Read the model definition and answer for the solid it produces. Units are mm, in the model's axes. A direction names the side the tool comes from. Coordinates: 2 decimals unless noted, no trailing zeros. Write each loop counter-clockwise with the first axis right and the second up, starting at its lowest first coordinate (ties: lowest second). Pieces come first, ordered by that corner, then holes.
1) The part is cut by section C-C (z = -9). Determine the outline of the cut face in (x, y), then the cut area to 3 significant figures.
2) Which of the six approach directions +Z, -Z, +X, -X, +Y, -Y give full straight-line access (tool end or side, diameter ignored) to faces 4 (the face through (30, 43, 0)), 5 (the face through (-35.18, 9.13, 0.96)), 6 (the face through (27.5, 163.4, -0.1))?
3) The part is cut by section A-A (y = 158). Determine the outline of the cut face in (x, z), then the cut area to 3 significant figures.
4) Find the intervals of material crossed by line 1 (Z direction, x = 37, y = 14); line 2 (X direction, y = 5.75, z = -25); line 3 (Y direction, x = 30.5, z = -20.5), in increasing order.
5) The part is cut by section D-D (x = -37). Determine the outline of the cut face in (y, z), then the cut area to 3 significant figures.
6) Determine the mould class of faces 1 (the face through (-32.5, 121, 0)), 2 (the face through (34, 18, 0)), 3 (the face through (25.4, 153.76, 0.17)) for opening direction X: +X half, -X half, draft (parallel to the pull), parting line (faces both ways), or undercut.
7) The part is cut by section B-B (x = 37.5). Determine the outline of the cut face in (y, z).
8) Each of these flat-tipped pins is pushed along its axis until it touches: pin 1 Ø8 at (x, z) = (37.5, 0) entering from -Y; pin 2 Ø5 at (y, z) = (72.5, 22.5) entering from +X; pin 3 Ø25 at (y, z) = (32.5, 0) entering from +X; pin 4 Ø6 at (x, z) = (-37.5, -25) entering from -Y. Where does it stop, or does it pass through?
from build123d import *

# Parameters (mm, degrees)
SKIZZE1_W                            = 90
SKIZZE1_H                            = 172
AUFSATZ_LINEAR_AUSTRAGEN1_DEPTH      = 65
SKIZZE2_W                            = 15
SKIZZE2_H                            = 154
SCHNITT_LINEAR_AUSTRAGEN1_DEPTH      = 190.298705754
SKIZZE3_W                            = 65
SKIZZE3_H                            = 104
AUFSATZ_LINEAR_AUSTRAGEN2_DEPTH      = 2.5
SKIZZE4_W                            = 15
SKIZZE4_H                            = 154
SCHNITT_LINEAR_AUSTRAGEN2_DEPTH      = 190.298705754
SKIZZE5_W                            = 65
SKIZZE5_H                            = 104
AUFSATZ_LINEAR_AUSTRAGEN3_DEPTH      = 2.5
F_6_6_6_6_DURCHMESSER_BOHRUNG1_D     = 6.6
F_6_6_6_6_DURCHMESSER_BOHRUNG1_DEPTH = 172
BOHRUNG1_D                           = 5.02
BOHRUNG1_DEPTH                       = 172
F_6_6_6_6_DURCHMESSER_BOHRUNG2_D     = 6.6
BOHRUNG2_D                           = 5.02
F_5_0_5_DURCHMESSER_BOHRUNG1_D       = 5
F_5_0_5_DURCHMESSER_BOHRUNG1_DEPTH   = 17
F_5_0_5_DURCHMESSER_BOHRUNG1_TIP     = 1.502151548


with BuildPart() as part:
    # Skizze1 → Aufsatz-Linear austragen1 (new body)
    with BuildSketch(Plane(origin=(0, 0, -32.5), x_dir=(-1, 0, 0), z_dir=(0, 0, -1))):
        with Locations((0, 86)):
            Rectangle(SKIZZE1_W, SKIZZE1_H)
    extrude(amount=-AUFSATZ_LINEAR_AUSTRAGEN1_DEPTH)

    # Skizze2 → Schnitt-Linear austragen1 (cut, through all)
    with BuildSketch(Plane.XY.offset(32.5)):
        with Locations((-37.5, 95)):
            Rectangle(SKIZZE2_W, SKIZZE2_H)
    extrude(amount=-SCHNITT_LINEAR_AUSTRAGEN1_DEPTH, mode=Mode.SUBTRACT)

    # Skizze3 → Aufsatz-Linear austragen2 (add)
    with BuildSketch(Plane.ZY.offset(30)):
        with Locations((0, 120)):
            Rectangle(SKIZZE3_W, SKIZZE3_H)
    extrude(amount=AUFSATZ_LINEAR_AUSTRAGEN2_DEPTH)

    # Skizze4 → Schnitt-Linear austragen2 (cut, through all)
    with BuildSketch(Plane.XY.offset(32.5)):
        with Locations((37.5, 95)):
            Rectangle(SKIZZE4_W, SKIZZE4_H)
    extrude(amount=-SCHNITT_LINEAR_AUSTRAGEN2_DEPTH, mode=Mode.SUBTRACT)

    # Skizze5 → Aufsatz-Linear austragen3 (add)
    with BuildSketch(Plane(origin=(30, 0, 0), x_dir=(0, 0, -1), z_dir=(1, 0, 0))):
        with Locations((0, 120)):
            Rectangle(SKIZZE5_W, SKIZZE5_H)
    extrude(amount=AUFSATZ_LINEAR_AUSTRAGEN3_DEPTH)

    # Ø6.6 (6.6) Durchmesser Bohrung1
    with Locations(Plane(origin=(0, 0, 0), x_dir=(-1, 0, 0), z_dir=(0, -1, 0))):
        with Locations((37.5, -25), (37.5, 25)):
            Hole(F_6_6_6_6_DURCHMESSER_BOHRUNG1_D / 2, depth=F_6_6_6_6_DURCHMESSER_BOHRUNG1_DEPTH)

    # Bohrung1
    with Locations(Plane(origin=(0, 0, 0), x_dir=(-1, 0, 0), z_dir=(0, -1, 0))):
        with Locations((37.5, 0)):
            Hole(BOHRUNG1_D / 2, depth=BOHRUNG1_DEPTH)

    # Ø6.6 (6.6) Durchmesser Bohrung2 (through all)
    with Locations(Plane(origin=(0, 18, 0), x_dir=(1, 0, 0), z_dir=(0, 1, 0))):
        with Locations((37.5, 25), (37.5, -25)):
            Hole(F_6_6_6_6_DURCHMESSER_BOHRUNG2_D / 2)

    # Bohrung2 (through all)
    with Locations(Plane(origin=(0, 18, 0), x_dir=(1, 0, 0), z_dir=(0, 1, 0))):
        with Locations((37.5, 0)):
            Hole(BOHRUNG2_D / 2)

    # Ø5.0 (5) Durchmesser Bohrung1
    with Locations(Plane(origin=(0, 172, 0), x_dir=(1, 0, 0), z_dir=(0, 1, 0))):
        with Locations((-25, 0), (25, 0), (0, 25), (0, -25)):
            Hole(F_5_0_5_DURCHMESSER_BOHRUNG1_D / 2, depth=F_5_0_5_DURCHMESSER_BOHRUNG1_DEPTH)
            with Locations((0, 0, -(F_5_0_5_DURCHMESSER_BOHRUNG1_DEPTH + F_5_0_5_DURCHMESSER_BOHRUNG1_TIP / 2))):  # 118° drill point
                Cone(0, F_5_0_5_DURCHMESSER_BOHRUNG1_D / 2, F_5_0_5_DURCHMESSER_BOHRUNG1_TIP, mode=Mode.SUBTRACT)


solid = part.part
Reported:
1. outline: (-45, 0) - (45, 0) - (45, 18) - (30, 18) - (30, 68) - (32.5, 68) - (32.5, 172) - (-32.5, 172) - (-32.5, 68) - (-30, 68) - (-30, 18) - (-45, 18) - close
1. area: 11,400 mm2
2. face 4: +Z, -Z, +X
2. face 5: +Y, -Y
2. face 6: +Y
3. outline: (-32.5, -32.5) - (32.5, -32.5) - (32.5, 32.5) - (-32.5, 32.5) - close; hole circle Ø5 at (-25, 0); hole circle Ø5 at (0, -25); hole circle Ø5 at (0, 25); hole circle Ø5 at (25, 0)
3. area: 4,150 mm2
4. line 1: z = -32.5 to -28.26, -21.74 to -2.46, 2.46 to 21.74, 28.26 to 32.5
4. line 2: x = -45 to -40.8, -34.2 to 34.2, 40.8 to 45
4. line 3: y = 0 to 18, 68 to 172
5. outline: (0, -32.5) - (18, -32.5) - (18, -28.26) - (0, -28.26) - close; (0, -21.74) - (18, -21.74) - (18, -2.46) - (0, -2.46) - close; (0, 2.46) - (18, 2.46) - (18, 21.74) - (0, 21.74) - close; (0, 28.26) - (18, 28.26) - (18, 32.5) - (0, 32.5) - close
5. area: 847 mm2
6. face 1: -X half
6. face 2: draft
6. face 3: undercut
7. outline: (0, -32.5) - (18, -32.5) - (18, -28.3) - (0, -28.3) - close; (0, -21.7) - (18, -21.7) - (18, -2.51) - (0, -2.51) - close; (0, 2.51) - (18, 2.51) - (18, 21.7) - (0, 21.7) - close; (0, 28.3) - (18, 28.3) - (18, 32.5) - (0, 32.5) - close
8. pin 1: stops at y = 0
8. pin 2: stops at x = 32.5
8. pin 3: stops at x = 30
8. pin 4: passes through
